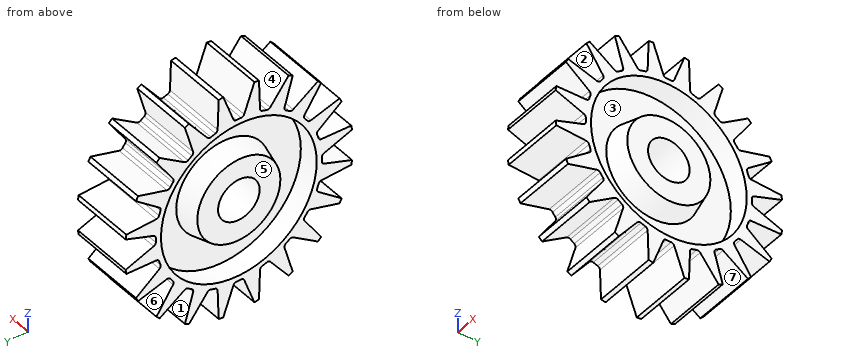
```python
from build123d import *

# Parameters (mm, degrees)
F3_DEPTH = 3
F4_COUNT = 20


with BuildPart() as f1:
    # F0 (on Front) → F1 (revolve)
    with BuildSketch(Plane.XZ):
        Polygon((3, 11), (0, 11), (-3, 11), (-3, 7.5), (-1, 7.5), (-1, 4.5), (-3, 4), (-3, 2), (0, 2), (3, 2), (3, 4), (1, 4.5), (1, 7.5), (3, 7.5), align=None)
    revolve(axis=Axis((-1.5, 0, 0), (1, 0, 0)))

    # F2 (on Right) → F3 (cut, symmetric)
    with BuildSketch(Plane.YZ):
        with BuildLine():
            ThreePointArc((-0.2257569502, 7.996813978), (0, 8), (0.2257569502, 7.996813978))
            ThreePointArc((0.2257569502, 7.996813978), (0.4028108647, 8.0485451993), (0.516130622, 8.1940884592))
            Line((0.516130622, 8.1940884592), (1.5, 10.8972473589))
            ThreePointArc((1.5, 10.8972473589), (0, 11), (-1.5, 10.8972473589))
            Line((-1.5, 10.8972473589), (-0.516130622, 8.1940884592))
            ThreePointArc((-0.516130622, 8.1940884592), (-0.4028108647, 8.0485451993), (-0.2257569502, 7.996813978))
        make_face()
    f3 = extrude(amount=F3_DEPTH, both=True, mode=Mode.SUBTRACT)

    # F4: F3 ×20 about axis
    f4_axis = Axis((3, 0, 0), (-1, 0, 0))
    for i in range(1, F4_COUNT):
        add(f3.rotate(f4_axis, i * 360 / F4_COUNT), mode=Mode.SUBTRACT)


solid = f1.part
```
Can you work these out from the model? Positions are in its coordinate system, mm. Face numbers are marked on the shaded views. A direction names the side the tool comes from. Give positions to 0.01 mm unless a question says otherwise; leave off trailing zeros. Order: outer loops, then holes, each group sorted by start corner. A loop starts at its lowest first (then second) coordinate and runs counter-clockwise, first axis right, second up. Notation, with made-up numbers: (9, 17) - (57, 17) arc R32 ccw to (57, 53) - close; hole circle Ø8 at (56.25, 35). An arc over 180 degrees is marked (long way). Use a Markdown table: item, result. Add a question column.
Q1. If we section it at D-D on z = -5.75: Write out the boundary of the cut face in (x, y).
Q2. On a 3-axis mill with a long thin cutter (end or side, diameter ignored), from which of +Z, -Z, +X, -X, +Y, -Y can I reach the whole of each face in a straight line? I mean the marked faces 1, 2, 3 and 4. Say none if no direction works.
Q3. If we mould it in two halves opening along Y, with no side actions, what happens to the marked faces 5, 6 and 7? For each: released by +Y, released by -Y, zero draft, split by the parting line, or undercut.
Q4. If we section it at A-A on x = -2.25: Count the separate pieces of the cut face and the enclosed holes in it, plus the area to 3 significant figures.
Q5. Please list where these lines run through material, in increasing order: line 1 along Z through (x, y) = (-2.05, 3); line 2 along Z through (x, y) = (1.85, -3); line 3 along Y through (x, z) = (-0.5, 9).
Q6. I'm going to push flat-ended pins straight in: pin 1 (5 mm diameter, centred on y = -5, z = 4.5, fed in from +X); pin 2 (3 mm diameter, centred on x = -2, z = -4, fed in from -Y). Where does each tip first touch, or does it pass through?
Q7. If we section it at B-B on z = 5.5: Write out the boundary of the cut face in (x, y), plus the area to 3 significant figures.
Answers follow:
| question | item | result |
|---|---|---|
| 1 | outline | (-3, -6.67) - (3, -6.67) - (3, -4.82) - (1, -4.82) - (1, 4.82) - (3, 4.82) - (3, 6.67) - (-3, 6.67) - (-3, 4.82) - (-1, 4.82) - (-1, -4.82) - (-3, -4.82) - close |
| 2 | face 1 | +X, -X |
| 2 | face 2 | +X, -X, -Y |
| 2 | face 3 | +X |
| 2 | face 4 | +Z, +X, -X |
| 3 | face 5 | zero draft |
| 3 | face 6 | released by +Y |
| 3 | face 7 | undercut |
| 4 | separate pieces | 2 |
| 4 | enclosed holes | 2 |
| 4 | area | 129 mm^2 |
| 5 | line 1 | z = -7.61 to -6.87, -2.99 to 2.99, 6.87 to 7.61 |
| 5 | line 2 | z = -7.61 to -6.87, -3.06 to 3.06, 6.87 to 7.61 |
| 5 | line 3 | y = -4.99 to -4.09, -2 to -0.81, 0.81 to 2, 4.09 to 4.99 |
| 6 | pin 1 | stops at x = 3 |
| 6 | pin 2 | stops at y = -9.9 |
| 7 | outline | (-3, -6.51) - (3, -6.51) - (3, -5.1) - (1, -5.1) - (1, 5.1) - (3, 5.1) - (3, 6.51) - (-3, 6.51) - (-3, 5.1) - (-1, 5.1) - (-1, -5.1) - (-3, -5.1) - close |
| 7 | area | 37.3 mm^2 |
